from build123d import *

# Parameters (mm, degrees)
SKETCH1_R           = 3.25
BOSS_EXTRUDE1_DEPTH = 22.686
SKETCH6_R           = 4.7
BOSS_EXTRUDE2_DEPTH = 8
FILLET2_R           = 0.75
SKETCH7_R           = 1.5
BOSS_EXTRUDE3_DEPTH = 1
BOSS_EXTRUDE4_DEPTH = 2


with BuildPart() as part:
    # Sketch1 → Boss-Extrude1 (new body)
    with BuildSketch(Plane(origin=(0, 0, 0), x_dir=(1, 0, 0), z_dir=(0, 1, 0))):
        Circle(SKETCH1_R)
    extrude(amount=BOSS_EXTRUDE1_DEPTH)

    # Sketch6 → Boss-Extrude2 (add)
    with BuildSketch(Plane(origin=(0, 22.686, 0), x_dir=(1, 0, 0), z_dir=(0, 1, 0))):
        Circle(SKETCH6_R)
    extrude(amount=BOSS_EXTRUDE2_DEPTH)

    # Fillet2
    fillet2_edges = [part.edges().sort_by_distance(p)[0] for p in [
        (-4.7, 30.686, 0),
    ]]
    fillet(fillet2_edges, radius=FILLET2_R)

    # Sketch7 → Boss-Extrude3 (add)
    with BuildSketch(Plane(origin=(0, 30.686, 0), x_dir=(1, 0, 0), z_dir=(0, 1, 0))):
        with Locations((-1.975, 0)):
            Circle(SKETCH7_R)
        with Locations((1.975, 0)):
            Circle(SKETCH7_R)
    extrude(amount=BOSS_EXTRUDE3_DEPTH)

    # Sketch8 → Boss-Extrude4 (add)
    with BuildSketch(Plane.XZ.offset(-22.686)):
        with BuildLine():
            Line((-1.016, 4.588871757), (-1.016, 6.620871757))
            Line((-1.016, 6.620871757), (1.016, 6.620871757))
            Line((1.016, 6.620871757), (1.016, 4.588871757))
            ThreePointArc((1.016, 4.588871757), (0, 4.7), (-1.016, 4.588871757))
        make_face()
        with BuildLine():
            Line((1.016, -6.620871757), (1.016, -4.588871757))
            ThreePointArc((1.016, -4.588871757), (0, -4.7), (-1.016, -4.588871757))
            Line((-1.016, -4.588871757), (-1.016, -6.620871757))
            Line((-1.016, -6.620871757), (1.016, -6.620871757))
        make_face()
    extrude(amount=-BOSS_EXTRUDE4_DEPTH)


solid = part.part
Read the model definition and answer for the solid it produces. Units are mm, in the model's axes. A direction names the side the tool comes from. Coordinates: 2 decimals unless noted, no trailing zeros. Write each loop counter-clockwise with the first axis right and the second up, starting at its lowest first coordinate (ties: lowest second). Pieces come first, ordered by that corner, then holes. Notation, with made-up numbers: (41, 68.5) -> (69, 68.5) arc R21 ccw to (69, 76.5) -> close; hole circle Ø4 at (21, 69). An arc over 180 degrees is marked (long way). Return JSON: item names as keys, results as strings.
(1) For a pull along X with two mould halves and no side action, classify faces 5 (the flat face through (1.016, 24, 6)), 6 (the cylindrical face through (-3.474, 31.179, -0.066)), 7 (the flat face through (-1.016, 24, -6)) as pulls with the +X half, pulls with the -X half, needs draft (parallel to the pull), parting line crosses it, or undercut.
Answers below:
{"face 5": "pulls with the +X half", "face 6": "undercut", "face 7": "pulls with the -X half"}
(2) The part is cut by section A-A on x = 0. Give the vertices of the cut face in (y, z).
Answers below:
{"outline": "(0, -3.25) -> (22.69, -3.25) -> (22.69, -6.62) -> (24.69, -6.62) -> (24.69, -4.7) -> (29.94, -4.7) arc R0.75 ccw to (30.69, -3.95) -> (30.69, 3.95) arc R0.75 ccw to (29.94, 4.7) -> (24.69, 4.7) -> (24.69, 6.62) -> (22.69, 6.62) -> (22.69, 3.25) -> (0, 3.25) -> close"}
(3) The part is cut by section C-C on z = 0. Give the vertices of the cut face in (x, y) (3 decimals).
Answers below:
{"outline": "(-4.7, 22.686) -> (-3.25, 22.686) -> (-3.25, 0) -> (3.25, 0) -> (3.25, 22.686) -> (4.7, 22.686) -> (4.7, 29.936) arc R0.75 ccw to (3.95, 30.686) -> (3.475, 30.686) -> (3.475, 31.686) -> (0.475, 31.686) -> (0.475, 30.686) -> (-0.475, 30.686) -> (-0.475, 31.686) -> (-3.475, 31.686) -> (-3.475, 30.686) -> (-3.95, 30.686) arc R0.75 ccw to (-4.7, 29.936) -> close"}
(4) Which of the six approach directions +Z, -Z, +X, -X, +Y, -Y give full straight-line access (tool end or side, diameter ignored) to faces 1 (the flat face through (-1.016, 24, 6)), 2 (the flat face through (1.016, 24, -6)), 3 (the cylindrical face through (3.406, 31.179, -0.451)), 4 (the cylindrical face through (-2.579, 11.184, 1.978))?
Answers below:
{"face 1": "+Z, -X, +Y, -Y", "face 2": "-Z, +X, +Y, -Y", "face 3": "+Y", "face 4": "-Y"}
(5) The part is cut by section D-D on y = 3. Give the vertices of the cut face in (x, z), then the cut area to 3 significant figures.
Answers below:
{"outline": "circle Ø6.5 at (0, 0)", "area": "33.2 mm^2"}
(6) Consider line 1 along Y through (x, z) = (-1.5, 2.75); line 2 along Y through (x, z) = (-3.75, -0.75); line 3 along X through (y, z) = (7, 0). Determine where each line is inside the solid, lowest interval first. Write a range as from..to.
Answers below:
{"line 1": "0..30.69", "line 2": "22.69..30.69", "line 3": "-3.25..3.25"}
(7) The part is cut by section B-B on y = 23. Give the vertices of the cut face in (x, z), then the cut area to 3 significant figures.
Answers below:
{"outline": "(-1.02, -6.62) -> (1.02, -6.62) -> (1.02, -4.59) arc R4.7 ccw to (1.02, 4.59) -> (1.02, 6.62) -> (-1.02, 6.62) -> (-1.02, 4.59) arc R4.7 ccw to (-1.02, -4.59) -> close", "area": "77.4 mm^2"}
(8) Each of these flat-tipped pins is pushed along its axis until it touches: P1, Ø0.6, axis at x = 0, z = 6, coming from the +Y side; P2, Ø3, axis at y = 10, z = -3.5, coming from the -X side; P3, Ø5, axis at x = -1, y = 11, coming from the -Z side. Where does it stop, or does it pass through?
Answers below:
{"P1": "y = 24.69", "P2": "x = -2.56", "P3": "z = -3.25"}
